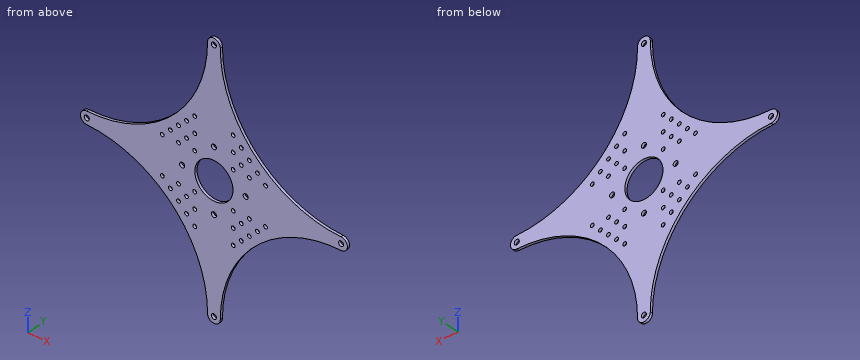
```python
from build123d import *

# Parameters (mm, degrees)
EXTRUDE_887_DEPTH           = 2
SKETCH_2_R                  = 2
CUT_EXTRUDE_1122_DEPTH      = 3
PATTERN_CIRCULAR_1192_COUNT = 4
SKETCH_4_R                  = 15
CUT_EXTRUDE_1537_DEPTH      = 3
SKETCH_5_R                  = 1.5
CUT_EXTRUDE_2052_DEPTH      = 3
PATTERN_CIRCULAR_2_COUNT    = 4


with BuildPart() as part:
    # Эскиз1 → Extrude 887 (new body)
    with BuildSketch(Plane(origin=(0, 0, 0), x_dir=(1, 0, 0), z_dir=(0, 1, 0))):
        with BuildLine():
            ThreePointArc((-5, 100), (0, 105), (5, 100))
            ThreePointArc((5, 100), (32.824855787, 32.824855787), (100, 5))
            ThreePointArc((100, 5), (105, 0), (100, -5))
            ThreePointArc((100, -5), (32.824855787, -32.824855787), (5, -100))
            ThreePointArc((5, -100), (0, -105), (-5, -100))
            ThreePointArc((-5, -100), (-32.824855787, -32.824855787), (-100, -5))
            ThreePointArc((-100, -5), (-105, 0), (-100, 5))
            ThreePointArc((-100, 5), (-32.824855787, 32.824855787), (-5, 100))
        make_face()
    extrude(amount=EXTRUDE_887_DEPTH)

    # Эскиз2 → Cut-Extrude 1122 (cut, through all)
    with BuildSketch(Plane(origin=(0, 2, 0), x_dir=(1, 0, 0), z_dir=(0, 1, 0))):
        with Locations((100, 0)):
            Circle(SKETCH_2_R)
        with Locations((25, 0)):
            Circle(SKETCH_2_R)
    cut_extrude_1122 = extrude(amount=-CUT_EXTRUDE_1122_DEPTH, mode=Mode.SUBTRACT)

    # Pattern Circular 1192: Cut-Extrude 1122 ×4 about axis
    pattern_circular_1192_axis = Axis((0, 0, 0), (0, 1, 0))
    for i in range(1, PATTERN_CIRCULAR_1192_COUNT):
        add(cut_extrude_1122.rotate(pattern_circular_1192_axis, i * 360 / PATTERN_CIRCULAR_1192_COUNT), mode=Mode.SUBTRACT)

    # Эскиз4 → Cut-Extrude 1537 (cut, through all)
    with BuildSketch(Plane(origin=(0, 2, 0), x_dir=(1, 0, 0), z_dir=(0, 1, 0))):
        Circle(SKETCH_4_R)
    extrude(amount=-CUT_EXTRUDE_1537_DEPTH, mode=Mode.SUBTRACT)

    # Эскиз5 → Cut-Extrude 2052 (cut, through all)
    with BuildSketch(Plane(origin=(0, 2, 0), x_dir=(1, 0, 0), z_dir=(0, 1, 0))):
        with Locations((40.60303038, 15.147186258)):
            Circle(SKETCH_5_R)
        with Locations((27.875108319, 15.147186258)):
            Circle(SKETCH_5_R)
        with Locations((21.511147288, 21.511147288)):
            Circle(SKETCH_5_R)
        with Locations((15.147186258, 15.147186258)):
            Circle(SKETCH_5_R)
        with Locations((15.147186258, 27.875108319)):
            Circle(SKETCH_5_R)
        with Locations((34.23906935, 21.511147288)):
            Circle(SKETCH_5_R)
        with Locations((27.875108319, 27.875108319)):
            Circle(SKETCH_5_R)
        with Locations((21.511147288, 34.23906935)):
            Circle(SKETCH_5_R)
        with Locations((15.147186258, 40.60303038)):
            Circle(SKETCH_5_R)
    cut_extrude_2052 = extrude(amount=-CUT_EXTRUDE_2052_DEPTH, mode=Mode.SUBTRACT)

    # Круговой массив2: Cut-Extrude 2052 ×4 about axis
    pattern_circular_2_axis = Axis((0, 0, 0), (0, 1, 0))
    for i in range(1, PATTERN_CIRCULAR_2_COUNT):
        add(cut_extrude_2052.rotate(pattern_circular_2_axis, i * 360 / PATTERN_CIRCULAR_2_COUNT), mode=Mode.SUBTRACT)


solid = part.part
```
Model file for the job. Use its own axes, mm. Give positions to 0.01 mm unless a question says otherwise; leave off trailing zeros. Order: outer loops, then holes, each group sorted by start corner. A loop starts at its lowest first (then second) coordinate and runs counter-clockwise, first axis right, second up.
1) Saw through at C-C, the plane z = 63. Write the cut outline in (x, y), then the cut area to 3 significant figures.
2) Wall check: probe 1 along Z at (x, y) = (-21, 0.25); probe 2 along Z at (x, y) = (-40, 1.5). Give the ranges that are in metal, low to high.
3) Pin check, flat tip, straight feed: pin 1 (5 mm diameter, centred on x = 15.15, z = -15.15, fed in from -Y). Stop position of the tip, or through.
4) Saw through at D-D, the plane y = 1.6. Count the separate pieces of the cut face and the enclosed holes in it, then the cut area to 3 significant figures.
5) Saw through at B-B, the plane x = 87. Write the cut outline in (y, z), then the cut area to 3 significant figures.
6) Saw through at A-A, the plane z = -9.5. Write the cut outline in (x, y).
Computed:
1. outline: (-12.5, 0) - (12.5, 0) - (12.5, 2) - (-12.5, 2) - close
1. area: 50.0 mm2
2. probe 1: z = -47.24 to -35.65, -32.83 to -22.92, -20.1 to 20.1, 22.92 to 32.83, 35.65 to 47.24
2. probe 2: z = -26.35 to -16.52, -13.77 to 13.77, 16.52 to 26.35
3. pin 1: stops at y = 0
4. separate pieces: 1
4. enclosed holes: 45
4. area: 10,700 mm2
5. outline: (0, -5.89) - (2, -5.89) - (2, 5.89) - (0, 5.89) - close
5. area: 23.6 mm2
6. outline: (-71.11, 0) - (-11.61, 0) - (-11.61, 2) - (-71.11, 2) - close; (11.61, 0) - (71.11, 0) - (71.11, 2) - (11.61, 2) - close
